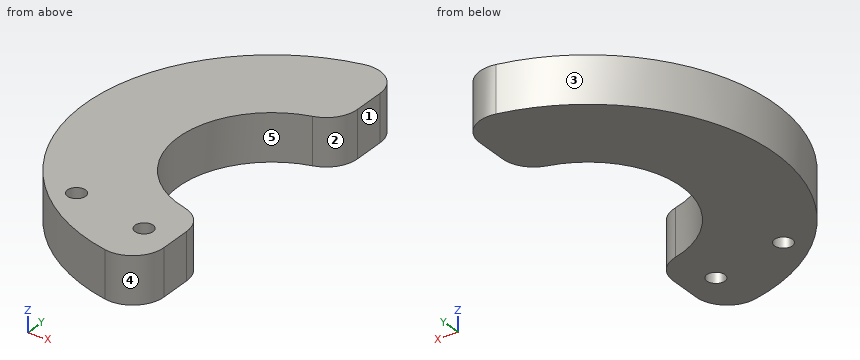
from build123d import *

# Parameters (mm, degrees)
FINGER_BODY_DEPTH      = 4.7625
SKETCH5_R              = 0.92075
FINGER_PIN_HOLES_DEPTH = 28.13612134


with BuildPart() as part:
    # Finger Drawing → Finger Body (new body)
    with BuildSketch(Plane.XY):
        with BuildLine():
            Line((0, 15.554259867), (0, 12.296722124))
            ThreePointArc((0, 12.296722124), (-0.664942107, 10.352439641), (-2.38125, 9.222541593))
            ThreePointArc((-2.38125, 9.222541593), (-9.525, 0), (-2.38125, -9.222541593))
            ThreePointArc((-2.38125, -9.222541593), (-0.664942107, -10.352439641), (0, -12.296722124))
            Line((0, -12.296722124), (0, -15.554259867))
            ThreePointArc((0, -15.554259867), (-1.166953686, -18.013604292), (-3.81, -18.66511184))
            ThreePointArc((-3.81, -18.66511184), (-19.05, 0), (-3.81, 18.66511184))
            ThreePointArc((-3.81, 18.66511184), (-1.166953686, 18.013604292), (0, 15.554259867))
        make_face()
    extrude(amount=FINGER_BODY_DEPTH)

    # Sketch5 → Finger Pin Holes (cut, through all)
    with BuildSketch(Plane.XY.offset(4.7625)):
        with Locations((-3.175, -13.930255965)):
            Circle(SKETCH5_R)
        with Locations((-11.1125, -12.4241527)):
            Circle(SKETCH5_R)
    extrude(amount=-FINGER_PIN_HOLES_DEPTH, mode=Mode.SUBTRACT)


solid = part.part
Could you check a few things on this model? Use its own coordinates, in mm. Face numbers are marked on the shaded views. A direction names the side the tool comes from. Coordinates: 2 decimals unless noted, no trailing zeros. Loops run counter-clockwise (first coordinate to the right, second up) from the corner with the lowest first, then second, coordinate; pieces in that order, holes last. Notation, with made-up numbers: (-35.5, -21.5) -> (5.5, -21.5) arc R37 ccw to (5.5, 16.5) -> close; hole circle Ø2 at (38, 15). An arc over 180 degrees is marked (long way). Answer in a Markdown table with one row per item.
(1) Imagine slicing it at B-B (z = 0.5). Give the number of separate pieces and of enclosed holes in the cut face, plus the area to 3 significant figures.
Results found:
| item | result |
|---|---|
| separate pieces | 1 |
| enclosed holes | 2 |
| area | 414 mm^2 |
(2) Imagine slicing it at D-D (x = -9). List the corners of the cut face in (y, z) for me, plus the area to 3 significant figures.
Results found:
| item | result |
|---|---|
| outline | (-16.79, 0) -> (-3.12, 0) -> (-3.12, 4.76) -> (-16.79, 4.76) -> close; (3.12, 0) -> (16.79, 0) -> (16.79, 4.76) -> (3.12, 4.76) -> close |
| area | 130 mm^2 |
(3) Thinking about a two-plate mould opening in Y: for the marked faces 3, 4 and 5, which applies, released by +Y, released by -Y, zero draft, split by the parting line, or undercut?
Results found:
| item | result |
|---|---|
| face 3 | split by the parting line |
| face 4 | released by -Y |
| face 5 | undercut |
(4) Will these pins go through, and if not, where does the flat tip stop? pin 1 Ø1.1 at (x, y) = (-3.18, -13.93) entering from +Z; pin 2 Ø1.5 at (y, z) = (-3, 2) entering from +X.
Results found:
| item | result |
|---|---|
| pin 1 | passes through |
| pin 2 | stops at x = -8.76 |
(5) Imagine slicing it at A-A (x = -6). List the corners of the cut face in (y, z) for me.
Results found:
| item | result |
|---|---|
| outline | (-18.08, 0) -> (-7.4, 0) -> (-7.4, 4.76) -> (-18.08, 4.76) -> close; (7.4, 0) -> (18.08, 0) -> (18.08, 4.76) -> (7.4, 4.76) -> close |
(6) If I drill on probe 1 along Y at (x, z) = (-3.5, 3.7); probe 2 along Y at (x, z) = (-7, 0.75); probe 3 along Y at (x, z) = (-8.75, 4.3), over which ranges is the centre line in solid material (lowest first)?
Results found:
| item | result |
|---|---|
| probe 1 | y = -18.71 to -14.79, -13.07 to -8.86, 8.86 to 18.71 |
| probe 2 | y = -17.72 to -6.46, 6.46 to 17.72 |
| probe 3 | y = -16.92 to -3.76, 3.76 to 16.92 |
(7) Imagine slicing it at C-C (x = -3). List the corners of the cut face in (y, z) for me.
Results found:
| item | result |
|---|---|
| outline | (-18.72, 0) -> (-14.83, 0) -> (-14.83, 4.76) -> (-18.72, 4.76) -> close; (-13.03, 0) -> (-9.04, 0) -> (-9.04, 4.76) -> (-13.03, 4.76) -> close; (9.04, 0) -> (18.72, 0) -> (18.72, 4.76) -> (9.04, 4.76) -> close |
(8) For the marked faces 1 and 2, which set-ups out of +Z, -Z, +X, -X, +Y, -Y let a thin tool reach every point of the face, with its end or its side?
Results found:
| item | result |
|---|---|
| face 1 | +Z, -Z, +X, +Y, -Y |
| face 2 | +Z, -Z, +X |
